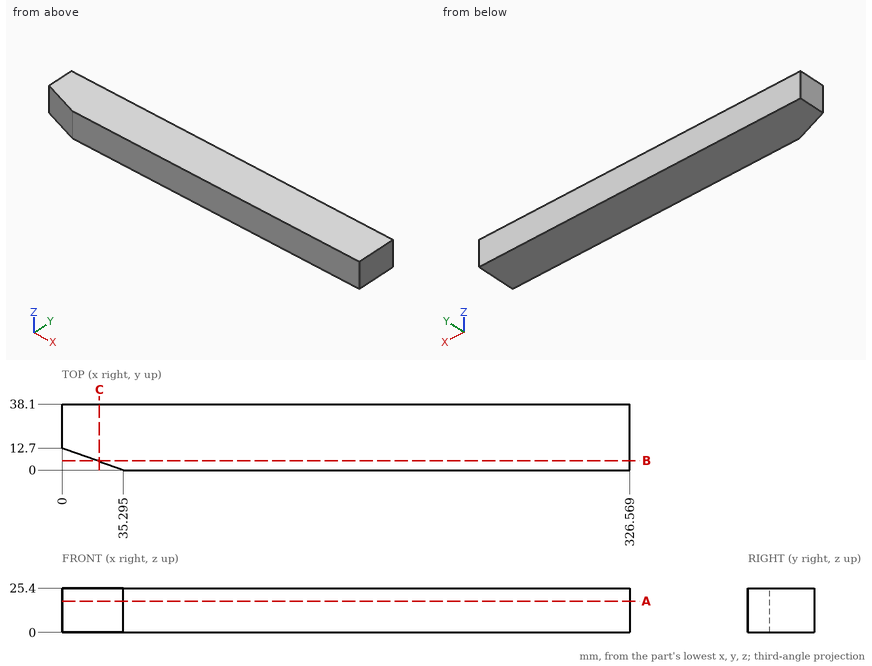
Source: three-view drawing plus pictorial views. Frame: mm from the lowest corner of the part. Give positions to 0.01 mm unless a question says otherwise; leave off trailing zeros. Order: outer loops, then holes, each group sorted by start corner. A loop starts at its lowest first (then second) coordinate and runs counter-clockwise, first axis right, second up. Notation, with made-up numbers: (61.25, -15.5) -> (81.25, -15.5) arc R17 cw to (81.25, 13.5) -> close; hole circle Ø10 at (33.25, 46.5). An arc over 180 degrees is marked (long way). Write each question's results on one line, items separated by ' | '. Start each with the question number.
Item 1: Line query: line 1 (Y direction, x = 25, z = 16.75) (1 decimal); line 2 (Y direction, x = 35, z = 17.25) (1 decimal). Output: solid intervals per line, ascending.
Item 2: Cut plane A-A on z = 18. Return the cut outline in (x, y) (1 decimal).
Item 3: Cut plane C-C on x = 21.5. Return the cut outline in (y, z).
Item 4: Cut plane B-B on y = 5.5. Return the cut outline in (x, z).
Established:
1) line 1: 3.7 to 38.1 | line 2: 0.1 to 38.1
2) outline: (0, 12.7) -> (35.3, 0) -> (326.6, 0) -> (326.6, 38.1) -> (0, 38.1) -> close
3) outline: (4.96, 0) -> (38.1, 0) -> (38.1, 25.4) -> (4.96, 25.4) -> close
4) outline: (20.01, 0) -> (326.57, 0) -> (326.57, 25.4) -> (20.01, 25.4) -> close
